Autodesk Inventor part; units mm, degrees
ref_plane "YZ Plane" through (0, 0, 0) normal (1, 0, 0) x (0, 1, 0)
ref_plane "XZ Plane" through (0, 0, 0) normal (0, 1, 0) x (-1, 0, 0)
ref_plane "XY Plane" through (0, 0, 0) normal (0, 0, 1) x (1, 0, 0)
sketch "Эскиз1" plane through (0, 0, 0) normal (0, 1, 0) x (-1, 0, 0)
  line L0 (200, 325) -> (-200, 325)
  line L1 (-200, 325) -> (-200, -325)
  line L2 (-200, -325) -> (200, -325)
  line L3 (200, -325) -> (200, 325)
  line L4 (200, 325) -> (-200, -325) construction
  line L5 (-200, 325) -> (200, -325) construction
  point P0 (0, 0)
  dimension "d0" = 650
  dimension "d1" = 400
extrude "Выдавливание1" add sketch "Эскиз1" along normal mid plane 6
fillet "Сопряжение1" radius 4 4 edges at (-200, 0, -325) (200, 0, -325) (200, 0, 325) (-200, 0, 325)
sketch "Эскиз3" plane through (0, 3, 0) normal (0, 1, 0) x (1, 0, 0)
  circle A0 centre (185, -105) radius 2
  arc A1 (-200, -321) -> (-196, -325) centre (-196, -321) ccw
  line L0 (-196, -325) -> (196, -325)
  arc A2 (196, -325) -> (200, -321) centre (196, -321) ccw
  line L1 (200, -321) -> (200, 321)
  arc A3 (200, 321) -> (196, 325) centre (196, 321) ccw
  line L2 (196, 325) -> (-196, 325)
  arc A4 (-196, 325) -> (-200, 321) centre (-196, 321) ccw
  line L3 (-200, 321) -> (-200, -321)
  line L4 (185, -413) -> (185, 413) construction
  circle A5 centre (-178, 315) radius 2
  line L5 (280, 0) -> (-280, 0) construction
  line L6 (-200, 315) -> (-183.7984, 315) construction
  circle A6 centre (-59.5, 315) radius 2
  circle A7 centre (59, 315) radius 2
  circle A8 centre (177.5, 315) radius 2
  circle A9 centre (185, -286.5) radius 2
  circle A10 centre (185, -233.5) radius 2
  circle A11 centre (185, -177) radius 2
  circle A12 centre (185, -124) radius 2
  circle A13 centre (-178, -315) radius 2
  circle A14 centre (-59.5, -315) radius 2
  circle A15 centre (59, -315) radius 2
  circle A16 centre (177.5, -315) radius 2
  line L7 (0, -50) -> (0, 50) construction
  circle A17 centre (-185, -105) radius 2
  circle A18 centre (-185, -286.5) radius 2
  circle A19 centre (-185, -233.5) radius 2
  circle A20 centre (-185, -177) radius 2
  circle A21 centre (185, 286.5) radius 2
  circle A22 centre (185, 233.5) radius 2
  circle A23 centre (185, 177) radius 2
  circle A24 centre (185, 124) radius 2
  circle A25 centre (-185, 286.5) radius 2
  circle A26 centre (-185, 233.5) radius 2
  circle A27 centre (-185, 177) radius 2
  circle A28 centre (-185, 119) radius 2
  circle A29 centre (185, -70) radius 2
  circle A30 centre (185, 75) radius 2
  circle A31 centre (185, 110) radius 2
  circle A32 centre (-185, -105) radius 2
  circle A33 centre (-185, -70) radius 2
  circle A34 centre (-185, 75) radius 2
  circle A35 centre (-185, 110) radius 2
  circle A36 centre (-185, -124) radius 2
  point P0 (0, 0)
  point P1 (185, 325)
  point P2 (185, -103)
  point P3 (185, -107)
  point P4 (185, -325)
  point P5 (0, 0)
  dimension "d7" = 4
  dimension "d15" = 4
  dimension "d17" = 220
  dimension "d34" = 10
  dimension "d35" = 22
  dimension "d38" = 118.5
  dimension "d43" = 4
  dimension "d44" = 38.5
  dimension "d45" = 4
  dimension "d46" = 4
  dimension "d47" = 4
  dimension "d48" = 53
  dimension "d49" = 53
  dimension "d50" = 56.5
  dimension "d51" = 100
  dimension "d58" = 35
  dimension "d59" = 35
  dimension "d60" = 14
extrude "Выдавливание3" cut sketch "Эскиз3" against normal up to surface (6 mm away) contours A0 | A5 | A6 | A7 | A8 | A9 | A10 | A11 | A12 | A13 | A14 | A15 | A16 | A17 | A18 | A19 | A20 | A21 | A22 | A23 | A24 | A25 | A26 | A27 | A28 | A29 | A30 | A31 | A33 | A34 | A35 | A36
sketch "Эскиз5" plane through (0, -3, 0) normal (0, -1, 0) x (1, 0, 0)
  circle A0 centre (148.4926, 47.4999) radius 1.5999
  circle A1 centre (115.4927, 47.5002) radius 1.6002
  circle A2 centre (82.4926, 47.4999) radius 1.5999
  circle A3 centre (82.4928, -47.4999) radius 1.6002
  circle A4 centre (115.4927, -47.5) radius 1.6001
  circle A5 centre (148.4927, -47.5) radius 1.6001
  circle A6 centre (-82.4927, 47.5) radius 1.5999
  circle A7 centre (-115.4927, 47.5) radius 1.6
  circle A8 centre (-148.4927, 47.4999) radius 1.5999
  circle A9 centre (-148.4927, -47.5) radius 1.6
  circle A10 centre (-115.4927, -47.5) radius 1.5999
  circle A11 centre (-82.4926, -47.5) radius 1.6
  point P0 (0, 0)
extrude "Выдавливание5" cut sketch "Эскиз5" against normal up to surface (6 mm away)
sketch "Эскиз6" plane through (0, -3, 0) normal (0, -1, 0) x (1, 0, 0)
  circle A0 centre (0, 60) radius 12.5
  circle A1 centre (0, -60) radius 12.5
  line L0 (0, 455) -> (0, -455) construction
  point P0 (0, 0)
  dimension "d61" = 25
  dimension "d62" = 25
  dimension "d63" = 60
  dimension "d64" = 60
extrude "Выдавливание6" cut sketch "Эскиз6" against normal up to surface (6 mm away)
sketch "Эскиз7" plane through (0, -3, 0) normal (0, -1, 0) x (1, 0, 0)
  line L0 (200, 321) -> (200, -321)
  line L1 (200, 0) -> (175, 0)
  line L2 (175, 0) -> (185, -17.3205)
  line L3 (185, -17.3205) -> (150, -17.3205)
  line L4 (150, -17.3205) -> (160, 0)
  line L5 (160, 0) -> (135, 0)
  line L6 (-200, -321) -> (-200, 321)
  line L7 (135, 0) -> (145, 17.3205)
  line L8 (145, 17.3205) -> (110, 17.3205)
  line L9 (110, 17.3205) -> (120, 0)
  line L10 (-280, 0) -> (280, 0) construction
  line L11 (101.6669, 0) -> (76.6669, 0)
  line L12 (76.6669, 0) -> (86.6669, -17.3205)
  line L13 (86.6669, -17.3205) -> (51.6669, -17.3205)
  line L14 (51.6669, -17.3205) -> (61.6669, 0)
  line L15 (61.6669, 0) -> (36.6669, 0)
  line L16 (36.6669, 0) -> (46.6669, 17.3205)
  line L17 (46.6669, 17.3205) -> (11.6669, 17.3205)
  line L18 (11.6669, 17.3205) -> (21.6669, 0)
  line L19 (3.3338, 0) -> (-21.6662, 0)
  line L20 (-21.6662, 0) -> (-11.6662, -17.3205)
  line L21 (-11.6662, -17.3205) -> (-46.6662, -17.3205)
  line L22 (-46.6662, -17.3205) -> (-36.6662, 0)
  line L23 (-36.6662, 0) -> (-61.6662, 0)
  line L24 (-61.6662, 0) -> (-51.6662, 17.3205)
  line L25 (-51.6662, 17.3205) -> (-86.6662, 17.3205)
  line L26 (-86.6662, 17.3205) -> (-76.6662, 0)
  line L27 (-94.9993, 0) -> (-119.9993, 0)
  line L28 (-119.9993, 0) -> (-109.9993, -17.3205)
  line L29 (-109.9993, -17.3205) -> (-144.9993, -17.3205)
  line L30 (-144.9993, -17.3205) -> (-134.9993, 0)
  line L31 (-134.9993, 0) -> (-159.9993, 0)
  line L32 (-159.9993, 0) -> (-149.9993, 17.3205)
  line L33 (-149.9993, 17.3205) -> (-184.9993, 17.3205)
  line L34 (-184.9993, 17.3205) -> (-174.9993, 0)
  line L35 (120, 0) -> (101.6669, 0)
  line L36 (-174.9993, 0) -> (-200, 0)
  line L37 (21.6669, 0) -> (3.3338, 0)
  line L38 (-76.6662, 0) -> (-94.9993, 0)
  point P0 (0, 0)
  dimension "d77" = 15
  dimension "d78" = 25
  dimension "d79" = 15
  dimension "d80" = 60
  dimension "d87" = 60
  dimension "d104" = 60
  dimension "d105" = 60
  dimension "d106" = 15
  dimension "d107" = 35
  dimension "d110" = 98.3331
split_face "Разделение2"
sketch "Эскиз8" plane through (-196, -3, 325) normal (0, -1, 0) x (1, 0, 0)
  circle A0 centre (381, -75) radius 3.1
  circle A1 centre (381, -45) radius 3.1
  circle A2 centre (381, -15) radius 3.1
  circle A3 centre (351, -15) radius 3.1
  circle A4 centre (11, -15) radius 3.1
  circle A5 centre (41, -15) radius 3.1
  circle A6 centre (11, -45) radius 3.1
  circle A7 centre (11, -75) radius 3.1
  point P0 (196, -325)
sketch "Эскиз9" plane through (-196, -3, -325) normal (0, -1, 0) x (1, 0, 0)
  circle A0 centre (381, 15) radius 3.1
  circle A1 centre (351, 15) radius 3.1
  circle A2 centre (381, 45) radius 3.1
  circle A3 centre (381, 75) radius 3.1
  circle A4 centre (41, 15) radius 3.1
  circle A5 centre (11, 15) radius 3.1
  circle A6 centre (11, 45) radius 3.1
  circle A7 centre (11, 75) radius 3.1
  point P0 (196, 325)
extrude "Выдавливание7" [suppressed]
extrude "Выдавливание8" [suppressed]
sketch "Эскиз10" plane through (-196, -3, 325) normal (0, -1, 0) x (1, 0, 0)
  circle A0 centre (68.41, -155.97) radius 1.59
  circle A1 centre (116.67, -157.51) radius 1.59
  circle A2 centre (83.61, -105.5) radius 1.55
  circle A3 centre (111.46, -105.5) radius 1.55
  circle A4 centre (68.29, -81.04) radius 1.59
  circle A5 centre (116.67, -74.54) radius 1.59
  circle A6 centre (146.01, -88.2899) radius 1.65
  circle A7 centre (177.0381, -104.4313) radius 1.65
  point P0 (196, -325)
extrude "Выдавливание9" [suppressed]
sketch "Эскиз11" plane through (-196, -3, -325) normal (0, -1, 0) x (1, 0, 0)
  circle A0 centre (121, 280) radius 3.15
  circle A1 centre (271, 280) radius 3.15
  circle A2 centre (121, 90) radius 3.15
  circle A3 centre (271, 90) radius 3.15
  point P0 (196, 325)
extrude "Выдавливание10" [suppressed]
sketch "Эскиз12" plane through (-196, -3, 325) normal (0, -1, 0) x (1, 0, 0)
  circle A0 centre (255, -10) radius 2
  circle A1 centre (136.5, -10) radius 2
  circle A2 centre (255, -640) radius 2
  circle A3 centre (136.5, -640) radius 2
  point P0 (196, -325)
extrude "Выдавливание11" [suppressed]
sketch "Эскиз14" plane through (-196, 3, 325) normal (0, 1, 0) x (1, 0, 0)
  circle A0 centre (11.994, 240.175) radius 2
  line L0 (-4, 325) -> (-4, 4)
  line L1 (-4, 325) -> (21.0007, 325)
  line L2 (11.994, 325) -> (11.994, 0) construction
  line L3 (21.0007, 325) -> (-4, 325)
  line L4 (0, 0) -> (392, 0)
  circle A1 centre (11.994, 189.852) radius 2
  point P0 (196, 325)
  dimension "d127" = 15.994
  dimension "d128" = 4
  dimension "d129" = 84.825
  dimension "d130" = 50.323
extrude "Выдавливание12" [suppressed]
sketch "Эскиз15" plane through (-196, 3, -325) normal (0, 1, 0) x (1, 0, 0)
  line L0 (33.816, 0) -> (33.816, -325) construction
  line L1 (392, 0) -> (0, 0)
  line L2 (21.0007, -325) -> (-4, -325)
  line L3 (-4, -4) -> (-4, -325)
  circle A0 centre (33.816, -78.112) radius 8.462
  circle A1 centre (33.816, -185.601) radius 8.462
  point P0 (196, -325)
  dimension "d133" = 37.816
  dimension "d134" = 16.924
  dimension "d135" = 139.399
  dimension "d136" = 107.489
extrude "Выдавливание13" [suppressed]
mirror "Зеркальное отражение1" [suppressed]
properties part number "platform"
Can you work these out from the model? Positions are in its coordinate system, mm. Round coordinates to 2 decimals unless told otherwise and drop trailing zeros. Write each loop counter-clockwise with the first axis right and the second up, starting at its lowest first coordinate (ties: lowest second). Pieces come first, ordered by that corner, then holes. Notation, with made-up numbers: (74.5, 42.25) -> (128.5, 42.25) arc R22 ccw to (128.5, 62.25) -> close; hole circle Ø9 at (44, -2.75). An arc over 180 degrees is marked (long way). One line per question, with ' | ' between items. Start each with the question number.
1) Suppose I cut it at A-A on z = 60. Write out the boundary of the cut face in (x, y).
2) Suppose I cut it at B-B on x = -5.5. Write out the boundary of the cut face in (y, z), then the cut area to 3 significant figures.
3) I need wall thicknesses on line 1 (Z direction, x = 59, y = -0.7); line 2 (Z direction, x = 0, y = 0); line 3 (X direction, y = 0.65, z = -75). Which ranges of each line are inside material? Lowest first, please. Write a range as [from, to].
4) If we mould it in two halves opening along Z, with no side actions, what happens to faces 1 (the flat face through (3, 3, 5)), 2 (the cylindrical face through (-1.627, -0.042, -47.606))? For each: released by +Z, released by -Z, zero draft, split by the parting line, or undercut.
Return value:
1) outline: (-200, -3) -> (-12.5, -3) -> (-12.5, 3) -> (-200, 3) -> close; (12.5, -3) -> (200, -3) -> (200, 3) -> (12.5, 3) -> close
2) outline: (-3, -325) -> (3, -325) -> (3, -71.22) -> (-3, -71.22) -> close; (-3, -48.78) -> (3, -48.78) -> (3, 48.78) -> (-3, 48.78) -> close; (-3, 71.22) -> (3, 71.22) -> (3, 325) -> (-3, 325) -> close | area: 3,630 mm2
3) line 1: z = [-325, -317], [-313, 313], [317, 325] | line 2: z = [-325, -72.5], [-47.5, 47.5], [72.5, 325] | line 3: x = [-200, -187], [-183, 183], [187, 200]
4) face 1: zero draft | face 2: undercut
